Check sheet for the modelled part. Datum: model origin and axes. Units: mm. Round coordinates to 2 decimals unless told otherwise and drop trailing zeros. Order: outer loops, then holes, each group sorted by start corner. A loop starts at its lowest first (then second) coordinate and runs counter-clockwise, first axis right, second up.
(1) Sectioned sample at B-B, the plane y = -38. Enter the section's corners in (x, z).
(2) Sectioned sample at C-C, the plane x = 289.5. Enter the section's corners in (y, z) (3 decimals).
(3) Sectioned sample at A-A, the plane z = -1. Enter the section's corners in (x, y).
(4) Thickness scan on probe 1 along Y at (x, z) = (186, -4); probe 2 along X at (y, z) = (-29.5, 30); probe 3 along Y at (x, z) = (-194, 32) (3 decimals). Record the ranges inside material, lowest first.
(5) Sectioned sample at D-D, the plane z = 28.5. Enter the section's corners in (x, y) (3 decimals), and give its area (3 significant figures).
(6) Depth check by flat-ended pin: pin 1 (1 mm diameter, centred on x = 67.5, y = -29, fed in from +Z). Enter the tip coordinate at first touch or a pass-through.
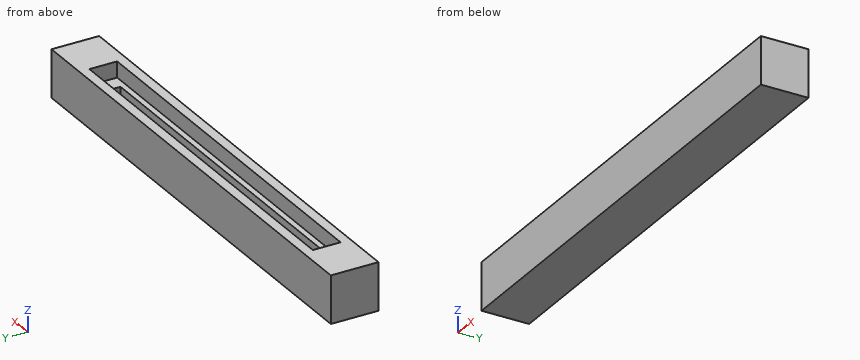
```python
from build123d import *

# Parameters (mm, degrees)
F0_W     = 762
F0_H     = 76.2
F1_DEPTH = 76.2
F2_W     = 609.6
F2_H     = 44.45
F3_DEPTH = 25.4
F4_W     = 558.8
F4_H     = 25.4
F5_DEPTH = 25.4


with BuildPart() as f1:
    # F0 (on Front) → F1 (new body)
    with BuildSketch(Plane.XZ):
        Rectangle(F0_W, F0_H)
    extrude(amount=F1_DEPTH)

    # F2 (on face) → F3 (cut)
    with BuildSketch(Plane.XY.offset(38.1)):
        with Locations((0, -38.1)):
            Rectangle(F2_W, F2_H)
    extrude(amount=-F3_DEPTH, mode=Mode.SUBTRACT)

    # F4 (on face) → F5 (cut)
    with BuildSketch(Plane.XY.offset(12.7)):
        with Locations((0, -38.1)):
            Rectangle(F4_W, F4_H)
    extrude(amount=-F5_DEPTH, mode=Mode.SUBTRACT)


solid = f1.part
```
Derived:
1. outline: (-381, -38.1) - (381, -38.1) - (381, 38.1) - (304.8, 38.1) - (304.8, 12.7) - (279.4, 12.7) - (279.4, -12.7) - (-279.4, -12.7) - (-279.4, 12.7) - (-304.8, 12.7) - (-304.8, 38.1) - (-381, 38.1) - close
2. outline: (-76.2, -38.1) - (0, -38.1) - (0, 38.1) - (-15.875, 38.1) - (-15.875, 12.7) - (-60.325, 12.7) - (-60.325, 38.1) - (-76.2, 38.1) - close
3. outline: (-381, -76.2) - (381, -76.2) - (381, 0) - (-381, 0) - close; hole (-279.4, -50.8) - (279.4, -50.8) - (279.4, -25.4) - (-279.4, -25.4) - close
4. probe 1: y = -76.2 to -50.8, -25.4 to 0
4. probe 2: x = -381 to -304.8, 304.8 to 381
4. probe 3: y = -76.2 to -60.325, -15.875 to 0
5. outline: (-381, -76.2) - (381, -76.2) - (381, 0) - (-381, 0) - close; hole (-304.8, -60.325) - (304.8, -60.325) - (304.8, -15.875) - (-304.8, -15.875) - close
5. area: 31,000 mm2
6. pin 1: stops at z = -12.7
